Geometry check sheet. Reference: drawing and pictorial views, mm from the part's lowest x, y, z. A direction names the side the tool comes from. Coordinates: 2 decimals unless noted, no trailing zeros. Loops run counter-clockwise (first coordinate to the right, second up) from the corner with the lowest first, then second, coordinate; pieces in that order, holes last. Notation, with made-up numbers: (71, 53) -> (121, 53) arc R26 ccw to (121, 75) -> close; hole circle Ø9 at (12, 72.25). An arc over 180 degrees is marked (long way). Use CSV: the item, a comma, the result in double quotes.
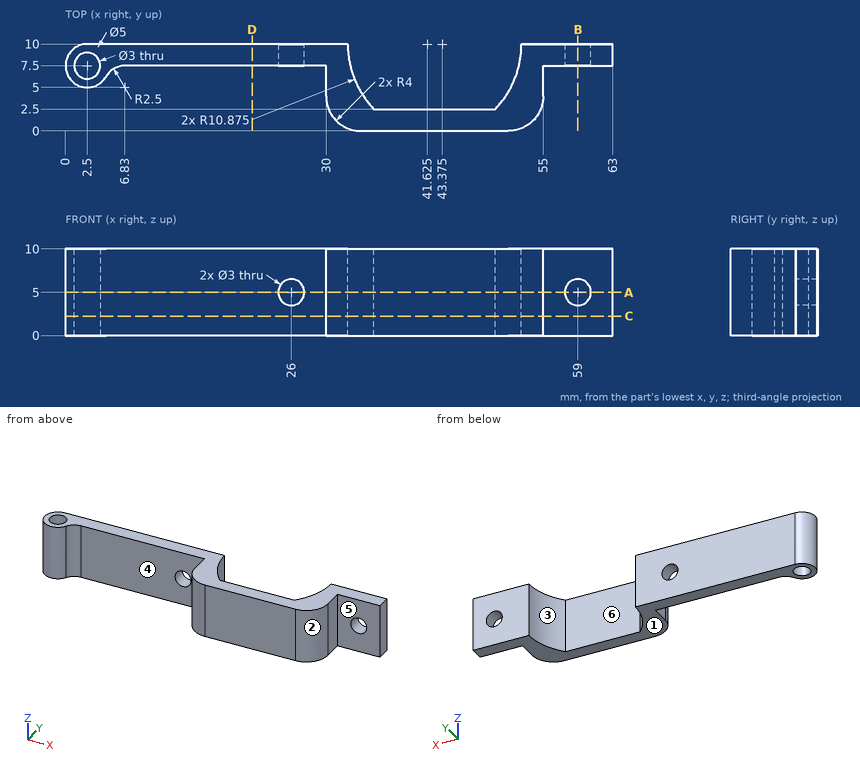
1) Cross-section at D-D on x = 21.5. Record the boundary of the cut face in (y, z).
Answer below:
outline,"(7.5, 0) -> (10, 0) -> (10, 10) -> (7.5, 10) -> close"
2) Cross-section at A-A on z = 5. Record the boundary of the cut face in (x, y) (3 decimals).
Answer below:
outline,"(2.5, 10) arc R2.5 ccw (long way) to (4.665, 6.25) arc R2.5 cw to (6.83, 7.5) -> (24.5, 7.5) -> (24.5, 10) -> close; (27.5, 7.5) -> (30, 7.5) -> (30, 4) arc R4 ccw to (34, 0) -> (51, 0) arc R4 ccw to (55, 4) -> (55, 7.5) -> (57.5, 7.5) -> (57.5, 10) -> (52.5, 10) arc R10.875 cw to (49.5, 2.5) -> (35.5, 2.5) arc R10.875 cw to (32.5, 10) -> (27.5, 10) -> close; (60.5, 7.5) -> (63, 7.5) -> (63, 10) -> (60.5, 10) -> close; hole circle Ø3 at (2.5, 7.5)"
3) Access from +Z, -Z, +X, -X, +Y, -Y to the whole of each face (thin tool, end or side, straight path). Record for the marked faces 4, 5 and 6.
Answer below:
face 4,"+Z, -Z, -Y"
face 5,"+Z, -Z, +X, -Y"
face 6,"+Z, -Z, +Y"
4) Cross-section at B-B on x = 59. Record the boundary of the cut face in (y, z), and give its area (3 significant figures).
Answer below:
outline,"(7.5, 0) -> (10, 0) -> (10, 3.5) -> (7.5, 3.5) -> close; (7.5, 6.5) -> (10, 6.5) -> (10, 10) -> (7.5, 10) -> close"
area,"17.5 mm²"
5) Draft check along X on the marked faces 1, 2 and 3. Enter one of: released by +X, released by -X, zero draft, split by the parting line, or undercut.
Answer below:
face 1,"zero draft"
face 2,"released by +X"
face 3,"undercut"
6) Cross-section at C-C on z = 2.25. Record the boundary of the cut face in (x, y) (3 decimals), and give its area (3 significant figures).
Answer below:
outline,"(2.5, 10) arc R2.5 ccw (long way) to (4.665, 6.25) arc R2.5 cw to (6.83, 7.5) -> (30, 7.5) -> (30, 4) arc R4 ccw to (34, 0) -> (51, 0) arc R4 ccw to (55, 4) -> (55, 7.5) -> (63, 7.5) -> (63, 10) -> (52.5, 10) arc R10.875 cw to (49.5, 2.5) -> (35.5, 2.5) arc R10.875 cw to (32.5, 10) -> close; hole circle Ø3 at (2.5, 7.5)"
area,"204 mm²"
7) Thickness scan on line 1 along Z through (x, y) = (26, 8.15); line 2 along X through (y, z) = (9.5, 8.5); line 3 along Y through (x, z) = (21, 6.5). Record the ranges inside material, lowest first. Write a range as from..to.
Answer below:
line 1,"z = 0..3.5, 6.5..10"
line 2,"x = 1..32.51, 52.49..63"
line 3,"y = 7.5..10"
8) Go/stop test with flat-tipped pins: pin 1 Ø1.5 at (y, z) = (5.5, 8) entering from -X (3 decimals); pin 2 Ø3 at (y, z) = (1.5, 3.5) entering from -X; pin 3 Ø2 at (y, z) = (5, 7.5) entering from +X. Record where each tip stops, or that it passes through.
Answer below:
pin 1,"stops at x = 0.335"
pin 2,"stops at x = 30.13"
pin 3,"stops at x = 55"
